For this review, take the finished solid that the model builds, in its own axes (mm). A direction names the side the tool comes from. Coordinates: 2 decimals unless noted, no trailing zeros. Order: outer loops, then holes, each group sorted by start corner. A loop starts at its lowest first (then second) coordinate and runs counter-clockwise, first axis right, second up. Notation, with made-up numbers: M -38.75,-24 L 10.25,-24 A31 cw 10.25,13 Z; hole C 9.5,45 d6. An arc over 180 degrees is marked long. Use one line per item in the form item = value. Start each with the question number.
```python
from build123d import *

# Parameters (mm, degrees)
F0_R          = 63.5
F1_DEPTH      = 63.5
F1_DEPTH_BACK = 63.5
F2_SIZE       = 10.16
F3_R          = 6.35
F4_R          = 52.5552622302
F5_DEPTH      = 45.72
F8_R          = 15.0932692433
F9_DEPTH      = 82.296
F10_R         = 5.08
F11_R         = 15.3989584518
F12_DEPTH     = 80.01
F13_R         = 5.08


# Not quite as in the source:
# - a fillet or chamfer that OpenCascade refuses, or shapes differently, is made with other operations: its cross-section is extruded or revolved along the edge and cut away or added


with BuildPart() as f1:
    # F0 (on Top) → F1 (new body, two sides)
    with BuildSketch(Plane.XY) as f1_sk:
        Circle(F0_R)
    extrude(amount=F1_DEPTH)
    extrude(f1_sk.sketch, amount=-F1_DEPTH_BACK)

    # F2
    f2_edges = [f1.edges().sort_by_distance(p)[0] for p in [
        (-63.5, 0, -63.5),
    ]]
    chamfer(f2_edges, length=F2_SIZE)

    # F3
    f3_edges = [f1.edges().sort_by_distance(p)[0] for p in [
        (-63.5, 0, 63.5),
    ]]
    fillet(f3_edges, radius=F3_R)

    # F4 (on face) → F5 (join)
    with BuildSketch(Plane.XY.offset(63.5)):
        Circle(F4_R)
    extrude(amount=F5_DEPTH)

    # F6: fillet of radius 45.9907683632 on 1 edges, made by hand


with BuildPart() as f6_tool2:
    # F6_s3 → F6_t4 (revolve)
    with BuildSketch(Plane.XZ):
        with BuildLine():
            ThreePointArc((52.5552622302, 63.2292316368), (39.0848780486, 95.7496158184), (6.564493867, 109.22))
            Line((6.564493867, 109.22), (52.5552622302, 109.22))
            Line((52.5552622302, 109.22), (52.5552622302, 63.2292316368))
        make_face()
    revolve(axis=Axis((0, 0, 109.22), (0, 0, 1)))

    split(bisect_by=Plane.XY.offset(63.5), keep=Keep.TOP)


with BuildPart() as f1_1:
    add(f1.part)

    # F6_t1: cut F6_tool2
    add(f6_tool2.part, mode=Mode.SUBTRACT)

    # F8 (on face) → F9 (join)
    with BuildSketch(Plane(origin=(0, 0, -63.5), x_dir=(1, 0, 0), z_dir=(0, 0, -1))):
        with Locations((26.5111289918, -24.0834727883)):
            Circle(F8_R)
    extrude(amount=F9_DEPTH)

    # F10
    f10_edges = [f1_1.edges().sort_by_distance(p)[0] for p in [
        (11.41786, 24.083473, -145.796),
    ]]
    fillet(f10_edges, radius=F10_R)

    # F11 (on face) → F12 (join)
    with BuildSketch(Plane(origin=(0, 0, -63.5), x_dir=(1, 0, 0), z_dir=(0, 0, -1))):
        with Locations((-18.4494890273, 5.414089188)):
            Circle(F11_R)
    extrude(amount=F12_DEPTH)

    # F13
    f13_edges = [f1_1.edges().sort_by_distance(p)[0] for p in [
        (-33.848447, -5.414089, -143.51),
    ]]
    fillet(f13_edges, radius=F13_R)


solid = f1_1.part
```
1. For pin 1 Ø12 at (x, y) = (-17.5, -25.5) entering from -Z; pin 2 Ø1 at (x, y) = (-24.5, 2) entering from -Z; pin 3 Ø6 at (x, y) = (-36, 37.5) entering from +Z, all flat-tipped, find the tip position at first contact; note any pin that passes through.
2. Consider section B-B, the plane z = -35. Write out the cut boundary in (x, y), plus the area to 3 significant figures.
3. Tool access review of faces 1 (the cylindrical face through (-13.77, -61.99, 2.68)), 2 (the cylindrical face through (15.39, 13.88, -101.57)), 3 (the flat face through (51, -17, 63.5)): name each direction out of +Z, -Z, +X, -X, +Y, -Y from which nothing blocks a thin tool from reaching the whole face with its end or side.
4. To check wall thickness, follow line 1 (Z direction, x = -30.5, y = 43); line 2 (Y direction, x = 39.5, z = -94.5); line 3 (X direction, y = 0, z = -117). State the ranges of each line that lie inside material, in increasing order.
5. Consider section A-A, the plane z = -82. Write out the cut boundary in (x, y), plus the area to 3 significant figures.
Answers follow:
q1.pin_1 = -141.81
q1.pin_2 = -143.51
q1.pin_3 = 81
q2.outline = C 0,0 d127
q2.area = 12,700 mm²
q3.face_1 = +Z, -Z
q3.face_2 = -Z
q3.face_3 = +Z
q4.line_1 = -63.5 to 63.5
q4.line_2 = 16.4 to 31.77
q4.line_3 = -32.87 to -4.03
q5.outline = C -18.45,-5.41 d30.8; C 26.51,24.08 d30.19
q5.area = 1,460 mm²
